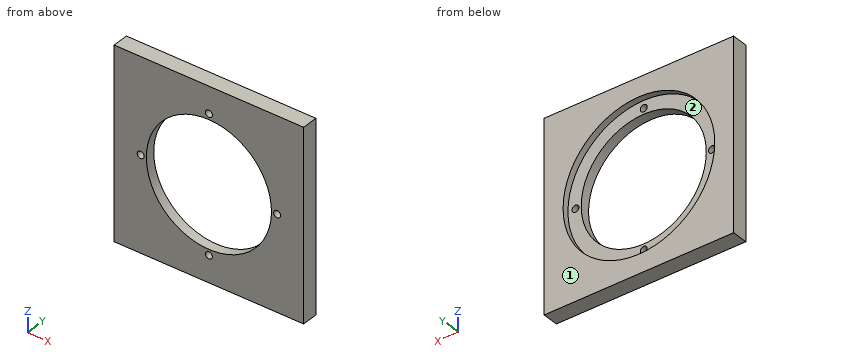
from build123d import *

# Parameters (mm, degrees)
SKETCH1_W               = 150
SKETCH1_H               = 150
SKETCH1_R               = 49.5
BOSS_EXTRUDE1_DEPTH     = 12.5984
SKETCH2_R               = 60
CUT_EXTRUDE1_DEPTH      = 5
CUT_EXTRUDE2_DEPTH      = 107.81160837
CUT_EXTRUDE2_DEPTH_BACK = 107.81160837
SKETCH3_R               = 2.75


with BuildPart() as part:
    # Sketch1 → Boss-Extrude1 (new body)
    with BuildSketch(Plane(origin=(0, 0, 0), x_dir=(1, 0, 0), z_dir=(0, 1, 0))):
        Rectangle(SKETCH1_W, SKETCH1_H)
        with Locations(Location((0, 0, 0), (0, 0, 270))):
            Circle(SKETCH1_R, mode=Mode.SUBTRACT)
    extrude(amount=-BOSS_EXTRUDE1_DEPTH)

    # Sketch2 → Cut-Extrude1 (cut)
    with BuildSketch(Plane(origin=(0, 0, 0), x_dir=(1, 0, 0), z_dir=(0, 1, 0))):
        with Locations(Location((0, 0, 0), (0, 0, 270))):
            Circle(SKETCH2_R)
    extrude(amount=-CUT_EXTRUDE1_DEPTH, mode=Mode.SUBTRACT)

    # Sketch3 → Cut-Extrude2 (cut, two sides: drawn at the far end of the back side and taken through both)
    with BuildSketch(Plane(origin=(0, 0, 0), x_dir=(1, 0, 0), z_dir=(0, 1, 0)).offset(-CUT_EXTRUDE2_DEPTH_BACK)):
        with Locations(Location((-54, 0, 0), (0, 0, 270))):
            Circle(SKETCH3_R)
        with Locations(Location((0, 54, 0), (0, 0, 270))):
            Circle(SKETCH3_R)
        with Locations(Location((54, 0, 0), (0, 0, 270))):
            Circle(SKETCH3_R)
        with Locations(Location((0, -54, 0), (0, 0, 270))):
            Circle(SKETCH3_R)
    extrude(amount=CUT_EXTRUDE2_DEPTH + CUT_EXTRUDE2_DEPTH_BACK, mode=Mode.SUBTRACT)


solid = part.part
Build history of the part. All positions in model axes, mm. Face numbers are marked on the shaded views. Coordinates: 2 decimals unless noted, no trailing zeros. Order: outer loops, then holes, each group sorted by start corner. A loop starts at its lowest first (then second) coordinate and runs counter-clockwise, first axis right, second up. Notation, with made-up numbers: M -29.75,-8 L 8.25,-8 A20 cw 8.25,21 Z; hole C -3,28 d10. An arc over 180 degrees is marked long. One line per question, with ' | ' between items. Start each with the question number.
Q1. Probe L1, parallel to X at y = -9.5, z = 0; L2, parallel to Z at x = -54, y = -8; L3, parallel to Y at x = -45, z = 38.5. List the from-to ranges inside material, lowest first. Write a range as from..to.
Q2. Saw through at B-B (y = -7.75). List the corners of the cut face in (x, z).
Q3. Saw through at C-C (x = 9). List the corners of the cut face in (y, z).
Q4. Saw through at D-D (z = 23). List the corners of the cut face in (x, y).
Q5. Flat gauge pins, fed straight in: pin 1 Ø9 at (x, z) = (0, 54) entering from +Y; pin 2 Ø4.5 at (x, z) = (0, -54) entering from +Y; pin 3 Ø7 at (x, z) = (-54, 0) entering from -Y. Where does each tip first touch, or does it go through?
Q6. Two-plate mould, pull along Z, no slides. Class the marked faces 1 and 2: +Z half, -Z half, draft (parallel to the pull), parting line (faces both ways), or undercut.
Q7. Saw through at A-A (z = 0). List the corners of the cut face in (x, y), then the cut area to 3 significant figures.
Check values:
1) L1: x = -75..-56.75, -51.25..-49.5, 49.5..51.25, 56.75..75 | L2: z = -75..-2.75, 2.75..75 | L3: y = -12.6..-5
2) outline: M -75,-75 L 75,-75 L 75,75 L -75,75 Z; hole C -54,0 d5.5; hole C 0,0 d99; hole C 0,-54 d5.5; hole C 0,54 d5.5; hole C 54,0 d5.5
3) outline: M -12.6,-75 L 0,-75 L 0,-59.32 L -5,-59.32 L -5,-48.67 L -12.6,-48.67 Z; M -12.6,48.67 L -5,48.67 L -5,59.32 L 0,59.32 L 0,75 L -12.6,75 Z
4) outline: M -75,-12.6 L -43.83,-12.6 L -43.83,-5 L -55.42,-5 L -55.42,0 L -75,0 Z; M 43.83,-12.6 L 75,-12.6 L 75,0 L 55.42,0 L 55.42,-5 L 43.83,-5 Z
5) pin 1: stops at y = -5 | pin 2: passes through | pin 3: stops at y = -12.6
6) face 1: draft | face 2: undercut
7) outline: M -75,-12.6 L -56.75,-12.6 L -56.75,-5 L -60,-5 L -60,0 L -75,0 Z; M -51.25,-12.6 L -49.5,-12.6 L -49.5,-5 L -51.25,-5 Z; M 49.5,-12.6 L 51.25,-12.6 L 51.25,-5 L 49.5,-5 Z; M 56.75,-12.6 L 75,-12.6 L 75,0 L 60,0 L 60,-5 L 56.75,-5 Z | area: 454 mm2
